from build123d import *

# Parameters (mm, degrees)
SKETCH1_W                = 114.3
SKETCH1_H                = 51.7398
BOSS_EXTRUDE1_DEPTH      = 6.35
M5_CLEARANCE_HOLE1_D     = 5.5
M5_CLEARANCE_HOLE1_DEPTH = 6.35
SKETCH6_W                = 16.51
SKETCH6_H                = 51.7398
BOSS_EXTRUDE2_DEPTH      = 19.05
SKETCH7_W                = 57.15
SKETCH7_H                = 51.7398
BOSS_EXTRUDE3_DEPTH      = 6.35
SKETCH10_R               = 10.9982
CUT_EXTRUDE1_DEPTH       = 6.35
M4_CLEARANCE_HOLE1_D     = 4.5
M4_CLEARANCE_HOLE1_DEPTH = 6.35


with BuildPart() as part:
    # Sketch1 → Boss-Extrude1 (new body)
    with BuildSketch(Plane(origin=(0, 0, 0), x_dir=(1, 0, 0), z_dir=(0, 1, 0))):
        Rectangle(SKETCH1_W, SKETCH1_H)
    extrude(amount=BOSS_EXTRUDE1_DEPTH)

    # M5 Clearance Hole1
    with Locations(Plane(origin=(0, 6.35, 0), x_dir=(1, 0, 0), z_dir=(0, 1, 0))):
        with Locations((25.4, 0), (-21.844, 0)):
            Hole(M5_CLEARANCE_HOLE1_D / 2, depth=M5_CLEARANCE_HOLE1_DEPTH)

    # Sketch6 → Boss-Extrude2 (add)
    with BuildSketch(Plane(origin=(0, 6.35, 0), x_dir=(1, 0, 0), z_dir=(0, 1, 0))):
        with Locations((-48.895, 0)):
            Rectangle(SKETCH6_W, SKETCH6_H)
    extrude(amount=BOSS_EXTRUDE2_DEPTH)

    # Sketch7 → Boss-Extrude3 (add)
    with BuildSketch(Plane(origin=(0, 25.4, 0), x_dir=(1, 0, 0), z_dir=(0, 1, 0))):
        with Locations((-28.575, 0)):
            Rectangle(SKETCH7_W, SKETCH7_H)
    extrude(amount=BOSS_EXTRUDE3_DEPTH)

    # Sketch10 → Cut-Extrude1 (cut)
    with BuildSketch(Plane(origin=(0, 31.75, 0), x_dir=(1, 0, 0), z_dir=(0, 1, 0))):
        with Locations((-21.844, 0)):
            Circle(SKETCH10_R)
    extrude(amount=-CUT_EXTRUDE1_DEPTH, mode=Mode.SUBTRACT)

    # M4 Clearance Hole1
    with Locations(Plane(origin=(0, 31.75, 0), x_dir=(1, 0, 0), z_dir=(0, 1, 0))):
        with Locations((-6.35, 15.494), (-37.338, 15.494), (-37.338, -15.494), (-6.35, -15.494)):
            Hole(M4_CLEARANCE_HOLE1_D / 2, depth=M4_CLEARANCE_HOLE1_DEPTH)


solid = part.part
Here's how the part is built. I have some questions about the finished solid (model axes, mm). A direction names the side the tool comes from. Coordinates: 2 decimals unless noted, no trailing zeros. Write each loop counter-clockwise with the first axis right and the second up, starting at its lowest first coordinate (ties: lowest second). Pieces come first, ordered by that corner, then holes.
Item 1: On a 3-axis mill with a long thin cutter (end or side, diameter ignored), from which of +Z, -Z, +X, -X, +Y, -Y can I reach the whole of each face in a straight line? I mean faces 1 (the flat face through (0, 29, 0)), 2 (the flat face through (8, 6.35, 0)), 3 (the cylindrical face through (-7.56, 28.531, 13.597)). Say none if no direction works.
Item 2: If I drill on line 1 (Z direction, x = -6.35, y = 29.5); line 2 (Y direction, x = -9.5, z = 2); line 3 (Z direction, x = -6, y = 28), over which ranges is the centre line in solid material (lowest first)?
Item 3: If we mould it in two halves opening along Z, with no side actions, what happens to faces 4 (the cylindrical face through (-35.09, 28.53, 15.4)), 5 (the flat face through (-14, 5, 25.87)), 6 (the flat face through (57.15, 3, 0))? For each: +Z half, -Z half, draft (parallel to the pull), parting line (faces both ways), or undercut.
Item 4: I want a section at D-D on z = 22.5. Write out the boundary of the cut face in (x, y), and give its area (3 significant figures).
Item 5: I want a section at B-B on x = 25.4. Write out the boundary of the cut face in (y, z).
Item 6: Will these pins go through, and if not, where does the flat tip stop? pin 1 (1.9 mm diameter, centred on y = 28, z = -3.5, fed in from +X); pin 2 (5 mm diameter, centred on x = 15.5, z = 15.5, fed in from +Y); pin 3 (1.5 mm diameter, centred on y = 22.5, z = -10.5, fed in from +X).
Item 7: I want a section at A-A on z = 0. Write out the boundary of the cut face in (x, y), and give its area (3 significant figures).
Item 8: I want a section at C-C on x = -6.35. Write out the boundary of the cut face in (y, z), and give its area (3 significant figures).
Findings below:
1. face 1: +Z, -Z, +X, +Y
1. face 2: +Z, -Z, +X
1. face 3: +Y
2. line 1: z = -25.87 to -17.74, -13.24 to 13.24, 17.74 to 25.87
2. line 2: y = 0 to 6.35, 25.4 to 31.75
2. line 3: z = -25.87 to -17.72, -13.27 to 13.27, 17.72 to 25.87
3. face 4: undercut
3. face 5: +Z half
3. face 6: draft
4. outline: (-57.15, 0) - (57.15, 0) - (57.15, 6.35) - (-40.64, 6.35) - (-40.64, 25.4) - (0, 25.4) - (0, 31.75) - (-57.15, 31.75) - close
4. area: 1,400 mm2
5. outline: (0, -25.87) - (6.35, -25.87) - (6.35, -2.75) - (0, -2.75) - close; (0, 2.75) - (6.35, 2.75) - (6.35, 25.87) - (0, 25.87) - close
6. pin 1: stops at x = 0
6. pin 2: stops at y = 6.35
6. pin 3: stops at x = -40.64
7. outline: (-57.15, 0) - (-24.59, 0) - (-24.59, 6.35) - (-40.64, 6.35) - (-40.64, 25.4) - (-32.84, 25.4) - (-32.84, 31.75) - (-57.15, 31.75) - close; (-19.09, 0) - (22.65, 0) - (22.65, 6.35) - (-19.09, 6.35) - close; (-10.85, 25.4) - (0, 25.4) - (0, 31.75) - (-10.85, 31.75) - close; (28.15, 0) - (57.15, 0) - (57.15, 6.35) - (28.15, 6.35) - close
7. area: 1,190 mm2
8. outline: (0, -25.87) - (6.35, -25.87) - (6.35, 25.87) - (0, 25.87) - close; (25.4, -25.87) - (31.75, -25.87) - (31.75, -17.74) - (25.4, -17.74) - close; (25.4, -13.24) - (31.75, -13.24) - (31.75, 13.24) - (25.4, 13.24) - close; (25.4, 17.74) - (31.75, 17.74) - (31.75, 25.87) - (25.4, 25.87) - close
8. area: 600 mm2
